```python
from build123d import *

# Parameters (mm, degrees)
SKETCH2_R           = 40
BOSS_EXTRUDE1_DEPTH = 100
SKETCH4_W           = 70
SKETCH4_H           = 4.556359802
CUT_EXTRUDE1_DEPTH  = 20
SKETCH5_W           = 70
SKETCH5_H           = 4.556359802
CUT_EXTRUDE2_DEPTH  = 20


with BuildPart() as part:
    # Sketch2 → Boss-Extrude1 (new, symmetric)
    with BuildSketch(Plane.XY):
        Circle(SKETCH2_R)
        with BuildLine():
            ThreePointArc((34.926090435, -2.273369064), (0, -35), (-34.926090435, -2.273369064))
            Line((-34.926090435, -2.273369064), (34.926090435, -2.273369064))
        make_face(mode=Mode.SUBTRACT)
        with BuildLine():
            Line((35, 2.278179901), (-35, 2.278179901))
            ThreePointArc((-35, 2.278179901), (0, 35.07406597), (35, 2.278179901))
        make_face(mode=Mode.SUBTRACT)
    extrude(amount=BOSS_EXTRUDE1_DEPTH, both=True)

    # Sketch4 → Cut-Extrude1 (cut)
    with BuildSketch(Plane.XY.offset(100)):
        Rectangle(SKETCH4_W, SKETCH4_H)
    extrude(amount=-CUT_EXTRUDE1_DEPTH, mode=Mode.SUBTRACT)

    # Sketch5 → Cut-Extrude2 (cut)
    with BuildSketch(Plane(origin=(0, 0, -100), x_dir=(-1, 0, 0), z_dir=(0, 0, -1))):
        Rectangle(SKETCH5_W, SKETCH5_H)
    extrude(amount=-CUT_EXTRUDE2_DEPTH, mode=Mode.SUBTRACT)


solid = part.part
```
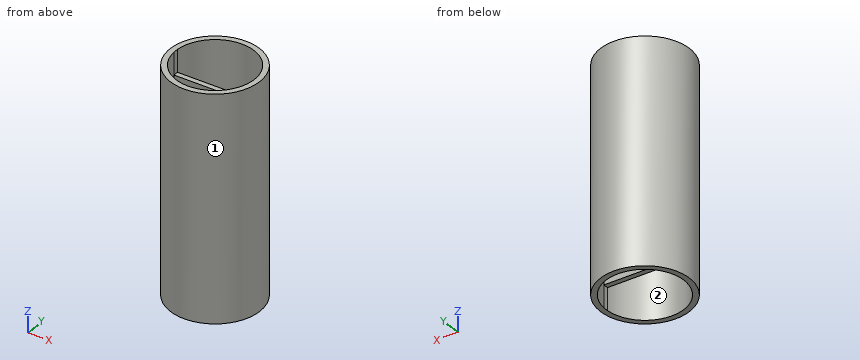
Geometry check sheet. Reference: the model listing, model coordinates, mm. Face numbers are marked on the shaded views. Coordinates: 2 decimals unless noted, no trailing zeros. Order: outer loops, then holes, each group sorted by start corner. A loop starts at its lowest first (then second) coordinate and runs counter-clockwise, first axis right, second up.
Q1. Draft check along X on the marked faces 1 and 2. Enter one of: released by +X, released by -X, zero draft, split by the parting line, or undercut.
Reply:
face 1: split by the parting line
face 2: undercut
Q2. Sectioned sample at A-A on x = 0. Record the cut outline in (y, z), and give its area (3 significant figures).
Reply:
outline: (-40, -100) - (-35, -100) - (-35, 100) - (-40, 100) - close; (-2.27, -80) - (2.28, -80) - (2.28, 80) - (-2.27, 80) - close; (35.07, -100) - (40, -100) - (40, 100) - (35.07, 100) - close
area: 2,710 mm2
Q3. Depth check by flat-ended pin: pin 1 Ø12 at (y, z) = (-3.5, -14.5) entering from +X; pin 2 Ø1.5 at (x, z) = (-15, -57.5) entering from -Y; pin 3 Ø4 at (y, z) = (-11, 78) entering from -X; pin 4 Ø5 at (x, y) = (7.5, -0.5) entering from -Z. Enter the tip coordinate at first touch or a pass-through.
Reply:
pin 1: stops at x = 40
pin 2: stops at y = -37.38
pin 3: stops at x = -38.97
pin 4: stops at z = -80
Q4. Sectioned sample at D-D on y = 0. Record the cut outline in (x, z), and give its area (3 significant figures).
Reply:
outline: (-40, -100) - (-35, -100) - (-35, -80) - (35, -80) - (35, -100) - (40, -100) - (40, 100) - (35, 100) - (35, 80) - (-35, 80) - (-35, 100) - (-40, 100) - close
area: 13,200 mm2
Q5. Thickness scan on probe 1 along Y at (x, z) = (-1.5, 33); probe 2 along Y at (x, z) = (-26, 35); probe 3 along X at (y, z) = (30.5, -25). Record the ranges inside material, lowest first.
Reply:
probe 1: y = -39.97 to -34.97, -2.27 to 2.28, 35.04 to 39.97
probe 2: y = -30.4 to -23.43, -2.27 to 2.28, 23.54 to 30.4
probe 3: x = -25.88 to -17.32, 17.32 to 25.88
Q6. Sectioned sample at B-B on y = -18.5. Record the cut outline in (x, z).
Reply:
outline: (-35.46, -100) - (-29.71, -100) - (-29.71, 100) - (-35.46, 100) - close; (29.71, -100) - (35.46, -100) - (35.46, 100) - (29.71, 100) - close
